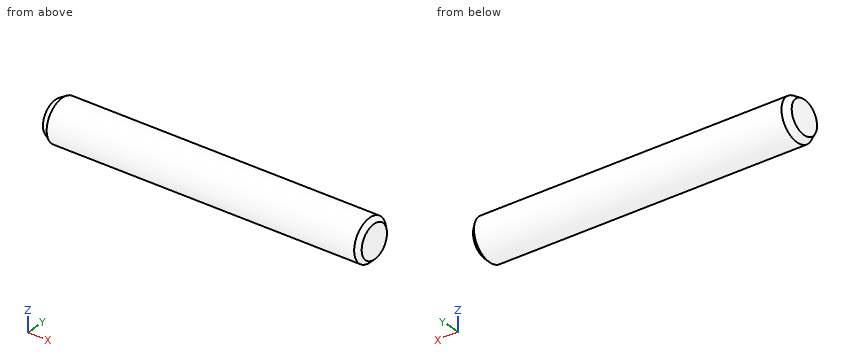
Autodesk Inventor part; units mm, degrees
ref_plane "Work Plane1" through (2.75, 0, 0) normal (0, -1, 0) x (1, 0, 0)
ref_plane "YZ Plane" through (0, 0, 0) normal (1, 0, 0) x (0, 1, 0)
ref_plane "XZ Plane" through (0, 0, 0) normal (0, 1, 0) x (-1, 0, 0)
sketch "Sketch1" plane through (0, 0, 0) normal (0, 0, 1) x (1, 0, 0)
  line L0 (20, 1.5) -> (20, 0)
  line L1 (-3, 0) -> (20, 0)
  line L2 (-7.6, 0) -> (24.6, 0)
  line L3 (0, 1.8) -> (0, -0.3)
  line L4 (-3, 1.5) -> (-3, 0)
  line L5 (8, 1.5) -> (8, 0) construction
  line L6 (-7.6, 0) -> (24.6, 0)
  line L7 (-3, 1.5) -> (20, 1.5)
  dimension "d4" = 3
  dimension "d5" = 20
  dimension "d6" = 12
  dimension "d13" = 3
revolve "Body" add sketch "Sketch1" angle 360 about axis through (-3, 0, 0) along (1, 0, 0)
thread "Thread1"
thread "Thread2"
chamfer "Chamfer1" distance 0.3077 distance2 0.3067 1 edges at (20, -1.5, 0) measured on face at (20, -0.7567, -0.3972)
chamfer "Chamfer2" distance 0.501 distance2 0.3067 1 edges at (-3, -1.5, 0) measured on face at (12.1288, 1.4951, -0.1207)
ref_plane "Work Plane1" through (2.75, 0, 0) normal (0, -1, 0) x (1, 0, 0)
equation "\"d4\" = KOH"
equation "\"d5\" = NLG"
equation "\"d6\" = GEL"
equation "\"d13\" = GD"
equation "\"d1\" = KOH"
equation "\"d7\" = GEL + GAL"
equation "\"d10\" = -0.5 * SPD + 0.5 * GD"
equation "\"d12\" = -0.5 * SPD + 0.5 * GD"
equation "\"NLG\" = 20"
equation "\"GEL\" = 12"
equation "\"GAL\" = 0.61345 * PTC"
equation "\"SPD\" = NND - 1.2269 * PTC"
equation "\"d0\" = GD"
equation "\"GUL\" = 0.61345 * PTC"
equation "\"KOH\" = NND"
equation "\"GD\" = NND"
equation "\"BDM\" = NND"
equation "\"GUL1\" = 0.5"
equation "\"GAL1\" = 0.5"
equation "\"d80\" = -GUL - GEL"
equation "\"d86\" = -KOH + GUL1"
equation "\"PTC\" = 0.5"
equation "\"THREADDIA\" = 3"
equation "\"TOA\" = 30deg"
equation "\"NND\" = 3"
equation "\"GD1\" = THREADDIA - 1.2269 * PTC"
properties part number "CSN 02 1174 - A M3 x 20" material "Steel, Mild"
Check sheet for the modelled part. Datum: model origin and axes. Units: mm. Coordinates: 2 decimals unless noted, no trailing zeros. Write each loop counter-clockwise with the first axis right and the second up, starting at its lowest first coordinate (ties: lowest second). Pieces come first, ordered by that corner, then holes.
Item 1: Scan lines: probe 1 along Z at (x, y) = (12.75, 0.1); probe 2 along Y at (x, z) = (-1.5, 0.8); probe 3 along Z at (x, y) = (1.5, 1.25). Record each from-to range of solid material in increasing order.
Numbers:
probe 1: z = -1.5 to 1.5
probe 2: y = -1.27 to 1.27
probe 3: z = -0.83 to 0.83
Item 2: Depth check by flat-ended pin: pin 1 Ø1.5 at (x, z) = (1.5, 1) entering from +Y; pin 2 Ø1.5 at (x, y) = (0, -1) entering from -Z. Enter the tip coordinate at first touch or a pass-through.
Numbers:
pin 1: stops at y = 1.48
pin 2: stops at z = -1.48
Item 3: Cross-section at A-A on x = 18.5. Record the boundary of the cut face in (y, z), then the cut area to 3 significant figures.
Numbers:
outline: circle Ø3 at (0, 0)
area: 7.07 mm2
